Input: dimensioned drawing with shaded views. Units: mm. Origin: part minimum x, y, z. A direction names the side the tool comes from. Round coordinates to 2 decimals unless told otherwise and drop trailing zeros. Order: outer loops, then holes, each group sorted by start corner. A loop starts at its lowest first (then second) coordinate and runs counter-clockwise, first axis right, second up.
Item 1: Reachability of the marked faces 1 and 2 from +Z, -Z, +X, -X, +Y, -Y: full face, straight path, thin tool, end or side. Return the list, or none.
Item 2: Cut plane B-B on z = 8. Output: boundary loops of the cut face in (x, y).
Item 3: Cut plane C-C on x = 14.4. Output: boundary loops of the cut face in (y, z), then the cut area to 3 significant figures.
Item 4: Cut plane A-A on y = 8. Output: boundary loops of the cut face in (x, z), then the cut area to 3 significant figures.
Item 5: Line query: L1, parallel to Y at x = 10.75, z = 1.25; L2, parallel to Y at x = 27.8, z = 12; L3, parallel to Z at x = 14.4, y = 1.05. Output: solid intervals per line, ascending.
Item 6: Cut plane D-D on y = 5. Output: boundary loops of the cut face in (x, z), then the cut area to 3 significant figures.
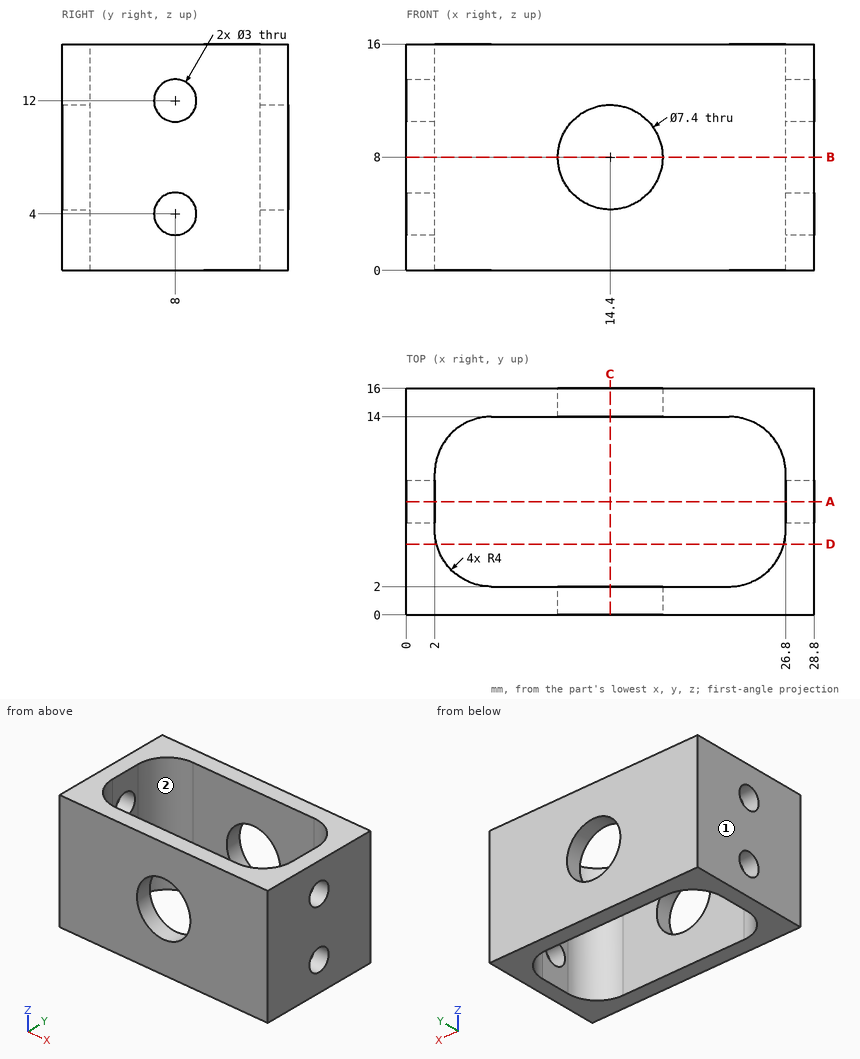
From the geometry:
1. face 1: +Z, -Z, -X, +Y, -Y
1. face 2: +Z, -Z
2. outline: (0, 0) - (10.7, 0) - (10.7, 2) - (6, 2) arc R4 cw to (2, 6) - (2, 10) arc R4 cw to (6, 14) - (10.7, 14) - (10.7, 16) - (0, 16) - close; (18.1, 0) - (28.8, 0) - (28.8, 16) - (18.1, 16) - (18.1, 14) - (22.8, 14) arc R4 cw to (26.8, 10) - (26.8, 6) arc R4 cw to (22.8, 2) - (18.1, 2) - close
3. outline: (0, 0) - (2, 0) - (2, 4.3) - (0, 4.3) - close; (0, 11.7) - (2, 11.7) - (2, 16) - (0, 16) - close; (14, 0) - (16, 0) - (16, 4.3) - (14, 4.3) - close; (14, 11.7) - (16, 11.7) - (16, 16) - (14, 16) - close
3. area: 34.4 mm2
4. outline: (0, 0) - (2, 0) - (2, 2.5) - (0, 2.5) - close; (0, 5.5) - (2, 5.5) - (2, 10.5) - (0, 10.5) - close; (0, 13.5) - (2, 13.5) - (2, 16) - (0, 16) - close; (26.8, 0) - (28.8, 0) - (28.8, 2.5) - (26.8, 2.5) - close; (26.8, 5.5) - (28.8, 5.5) - (28.8, 10.5) - (26.8, 10.5) - close; (26.8, 13.5) - (28.8, 13.5) - (28.8, 16) - (26.8, 16) - close
4. area: 40.0 mm2
5. L1: y = 0 to 2, 14 to 16
5. L2: y = 0 to 6.5, 9.5 to 16
5. L3: z = 0 to 4.3, 11.7 to 16
6. outline: (0, 0) - (2.13, 0) - (2.13, 16) - (0, 16) - close; (26.67, 0) - (28.8, 0) - (28.8, 16) - (26.67, 16) - close
6. area: 68.1 mm2
